Autodesk Inventor part; units mm, degrees
ref_plane "Midplane" through (0, -39, 16) normal (1, 0, 0) x (0, 0, -1)
ref_plane "YZ Plane" through (0, 0, 0) normal (1, 0, 0) x (0, 1, 0)
ref_plane "XZ Plane" through (0, 0, 0) normal (0, 1, 0) x (-1, 0, 0)
sketch "Sketch1" plane through (0, 0, 0) normal (0, 0, 1) x (1, 0, 0)
  line L0 (-67.5, -39) -> (67.5, -39)
  line L1 (67.5, -39) -> (67.5, 39)
  line L2 (67.5, 39) -> (-67.5, 39)
  line L3 (-67.5, 39) -> (-67.5, -39)
  point P0 (0, 0)
  point P1 (-67.5, 0)
  point P2 (0, 39)
  dimension "d0" = 78
  dimension "d1" = 135
extrude "Extrusion1" add sketch "Sketch1" along normal blind 12
sketch "Sketch2" plane through (0, 0, 12) normal (0, 0, 1) x (1, 0, 0)
  line L0 (67.5, -39) -> (-67.5, -39)
  line L1 (-67.5, 39) -> (67.5, 39)
  line L2 (-30.5, -39) -> (30.5, -39)
  line L3 (30.5, -39) -> (30.5, 39)
  line L4 (30.5, 39) -> (-30.5, 39)
  line L5 (-30.5, 39) -> (-30.5, -39)
  line L6 (0, 54.6) -> (0, -54.6)
  line L7 (-95.2, 0) -> (95.2, 0)
  dimension "d4" = 61
extrude "Extrusion2" add sketch "Sketch2" along normal blind 4
sketch "Sketch3" plane through (0, 0, 0) normal (0, 0, -1) x (-1, 0, 0)
  line L0 (67.5, -39) -> (-67.5, -39)
  line L1 (67.5, 39) -> (67.5, -39)
  line L2 (-67.5, 39) -> (67.5, 39)
  line L3 (23.5, -39) -> (-24.5, -39)
  line L4 (-24.5, -39) -> (-24.5, 39)
  line L5 (-24.5, 39) -> (23.5, 39)
  line L6 (23.5, 39) -> (23.5, -39)
  dimension "d8" = 48
  dimension "d9" = 44
extrude "Extrusion3" cut sketch "Sketch3" against normal blind 4 contours L0 L4 L2 L6
sketch "Sketch4" plane through (0, 0, 12) normal (0, 0, 1) x (1, 0, 0)
  line L0 (67.5, 39) -> (67.5, -39)
  line L1 (30.5, 39) -> (67.5, 39)
  line L2 (67.5, 0) -> (0.1063, 0) construction
  line L3 (-30.5, -39) -> (-30.5, 39)
  line L4 (30.5, -39) -> (-30.5, -39)
  line L5 (30.5, 39) -> (30.5, -39)
  line L6 (-30.5, 39) -> (30.5, 39)
  line L7 (-30.5, -39) -> (-30.5, 39)
  line L8 (-67.5, 39) -> (-30.5, 39)
  line L9 (-67.5, -39) -> (-67.5, 39)
  line L10 (-30.5, -39) -> (-67.5, -39)
  line L11 (0, 39) -> (0, 3.4704) construction
  point P0 (55.5, 27)
  point P1 (-55.5, 27)
  point P2 (-55.5, -27)
  point P3 (55.5, -27)
  dimension "d12" = 111
  dimension "d13" = 54
hole "Hole1" at (55.5, 27, 12) at (-55.5, 27, 12) at (-55.5, -27, 12) at (55.5, -27, 12) direction (0, 0, -1) diameter 10 depth 12
fillet "Fillet1" radius 12 4 edges at (67.5, 39, 6) (67.5, -39, 6) (-67.5, 39, 6) (-67.5, -39, 6)
ref_plane "Midplane" through (0, -39, 16) normal (1, 0, 0) x (0, 0, -1)
properties part number "Base Plate" material "Carbon Steel"
Geometry: final body of the model. Coordinates: model frame, mm. A direction names the side the tool comes from. Give positions to 0.01 mm unless a question says otherwise; leave off trailing zeros. Write each loop counter-clockwise with the first axis right and the second up, starting at its lowest first coordinate (ties: lowest second). Pieces come first, ordered by that corner, then holes. Notation, with made-up numbers: (-18, 44.5) -> (-14, 44.5) arc R22 ccw to (-14, 80.5) -> close; hole circle Ø11 at (-15.75, -35). An arc over 180 degrees is marked (long way). Answer in a Markdown table with one row per item.
(1) Section query D-D on y = -30.5. Return loops of the section in (x, z).
Answers below:
| item | result |
|---|---|
| outline | (-66.98, 0) -> (-59.07, 0) -> (-59.07, 12) -> (-66.98, 12) -> close; (-51.93, 0) -> (-23.5, 0) -> (-23.5, 4) -> (24.5, 4) -> (24.5, 0) -> (51.93, 0) -> (51.93, 12) -> (30.5, 12) -> (30.5, 16) -> (-30.5, 16) -> (-30.5, 12) -> (-51.93, 12) -> close; (59.07, 0) -> (66.98, 0) -> (66.98, 12) -> (59.07, 12) -> close |
(2) Section query A-A on z = 2. Return loops of the section in (x, y), then the cut area to 3 significant figures.
Answers below:
| item | result |
|---|---|
| outline | (-67.5, -27) arc R12 ccw to (-55.5, -39) -> (-23.5, -39) -> (-23.5, 39) -> (-55.5, 39) arc R12 ccw to (-67.5, 27) -> close; (24.5, -39) -> (55.5, -39) arc R12 ccw to (67.5, -27) -> (67.5, 27) arc R12 ccw to (55.5, 39) -> (24.5, 39) -> close; hole circle Ø10 at (-55.5, -27); hole circle Ø10 at (-55.5, 27); hole circle Ø10 at (55.5, -27); hole circle Ø10 at (55.5, 27) |
| area | 6,350 mm^2 |
(3) Section query C-C on x = -57. Return loops of the section in (y, z).
Answers below:
| item | result |
|---|---|
| outline | (-38.91, 0) -> (-31.77, 0) -> (-31.77, 12) -> (-38.91, 12) -> close; (-22.23, 0) -> (22.23, 0) -> (22.23, 12) -> (-22.23, 12) -> close; (31.77, 0) -> (38.91, 0) -> (38.91, 12) -> (31.77, 12) -> close |
(4) Pin query (flat end, axial travel): pin 1 (1.5 mm diameter, centred on y = -8.5, z = 13.5, fed in from +X); pin 2 (9 mm diameter, centred on x = 55.5, y = 27, fed in from +Z); pin 3 (16 mm diameter, centred on x = 55.5, y = -27, fed in from +Z); pin 4 (2 mm diameter, centred on y = 29.5, z = 8, fed in from -X). Return the tip coordinate at first contact, or that it passes through.
Answers below:
| item | result |
|---|---|
| pin 1 | x = 30.5 |
| pin 2 | through |
| pin 3 | z = 12 |
| pin 4 | x = -67.41 |
(5) Section query B-B on y = 16.5. Return loops of the section in (x, z).
Answers below:
| item | result |
|---|---|
| outline | (-67.5, 0) -> (-23.5, 0) -> (-23.5, 4) -> (24.5, 4) -> (24.5, 0) -> (67.5, 0) -> (67.5, 12) -> (30.5, 12) -> (30.5, 16) -> (-30.5, 16) -> (-30.5, 12) -> (-67.5, 12) -> close |
(6) Draft query along X for faces 1 (the flat face through (1, 1, 4)), 2 (the cylindrical face through (63.89, -35.58, 6.08)), 3 (the flat face through (49, 1, 12)). Return one class per face: +X half, -X half, draft (parallel to the pull), parting line (faces both ways), or undercut.
Answers below:
| item | result |
|---|---|
| face 1 | undercut |
| face 2 | +X half |
| face 3 | draft |
(7) Set-up query: faces 4 (the flat face through (0, 1, 16)), 5 (the cylindrical face through (64.08, 35.39, 6.08)), 6 (the flat face through (-30.5, 1, 14)), 7 (the flat face through (24.5, -1, 2)), 8 (the flat face through (30.5, -1, 14)). Return all of +Z, -Z, +X, -X, +Y, -Y with unobstructed straight access to the full face (end or side cutting, diameter ignored); none if empty.
Answers below:
| item | result |
|---|---|
| face 4 | +Z, +X, -X, +Y, -Y |
| face 5 | +Z, -Z, +X, +Y |
| face 6 | +Z, -X, +Y, -Y |
| face 7 | -Z, +Y, -Y |
| face 8 | +Z, +X, +Y, -Y |
(8) Ray query, line 1 along X through (y, z) = (-27, 8); line 2 along Y through (x, z) = (55.5, 9); line 3 along X through (y, z) = (-27, 3.5). Return the intervals inside material, ascending. Write a range as [from, to].
Answers below:
| item | result |
|---|---|
| line 1 | [-67.5, -60.5], [-50.5, 50.5], [60.5, 67.5] |
| line 2 | [-39, -32], [-22, 22], [32, 39] |
| line 3 | [-67.5, -60.5], [-50.5, -23.5], [24.5, 50.5], [60.5, 67.5] |
